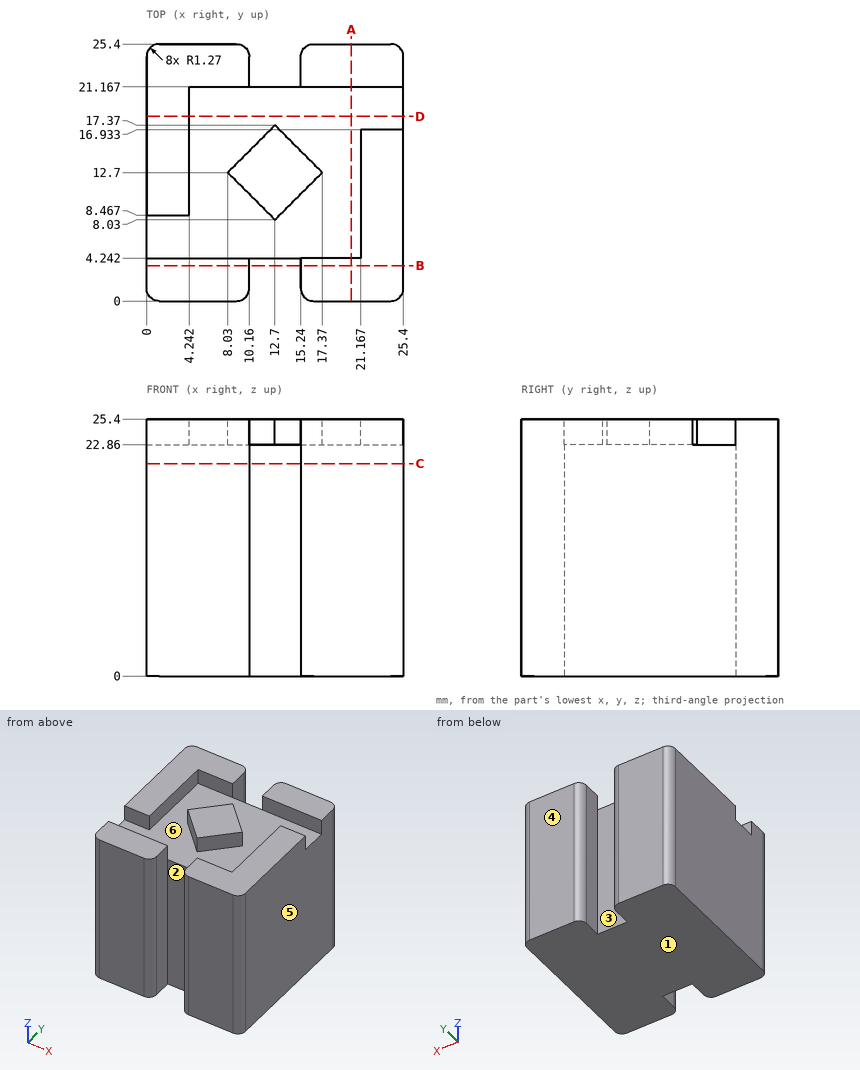
Print and shaded views of the part. All mm, measured from the part's lowest x, y and z. A direction names the side the tool comes from. Coordinates: 2 decimals unless noted, no trailing zeros. Order: outer loops, then holes, each group sorted by start corner. A loop starts at its lowest first (then second) coordinate and runs counter-clockwise, first axis right, second up. Notation, with made-up numbers: (51.5, 46) - (55.5, 46) arc R34 ccw to (55.5, 77) - close; hole circle Ø8 at (69.25, 13). An arc over 180 degrees is marked (long way). Put each result on its own line as item: value.
1. Saw through at C-C (z = 21). Write the cut outline in (x, y), and give its area (3 significant figures).
Answer sheet:
outline: (0, 1.27) arc R1.27 ccw to (1.27, 0) - (8.89, 0) arc R1.27 ccw to (10.16, 1.27) - (10.16, 4.24) - (15.24, 4.24) - (15.24, 1.27) arc R1.27 ccw to (16.51, 0) - (24.13, 0) arc R1.27 ccw to (25.4, 1.27) - (25.4, 24.13) arc R1.27 ccw to (24.13, 25.4) - (16.51, 25.4) arc R1.27 ccw to (15.24, 24.13) - (15.24, 21.17) - (10.16, 21.17) - (10.16, 24.13) arc R1.27 ccw to (8.89, 25.4) - (1.27, 25.4) arc R1.27 ccw to (0, 24.13) - close
area: 599 mm^2
2. Drop flat-ended pins along their axis: P1, Ø0.8, axis at x = 2.5, z = 24.5, coming from the -Y side; P2, Ø1.5, axis at x = 8, y = 14.5, coming from the +Z side; P3, Ø0.8, axis at y = 17.5, z = 24.5, coming from the +X side; P4, Ø4, axis at x = 13, z = 8, coming from the -Y side. Give the stop position or say it passes through.
Answer sheet:
P1: stops at y = 0
P2: stops at z = 22.86
P3: stops at x = 12.97
P4: stops at y = 4.24
3. Saw through at D-D (y = 18.25). Write the cut outline in (x, z), and give its area (3 significant figures).
Answer sheet:
outline: (0, 0) - (25.4, 0) - (25.4, 22.86) - (4.24, 22.86) - (4.24, 25.4) - (0, 25.4) - close
area: 591 mm^2
4. Saw through at A-A (x = 20.25). Write the cut outline in (y, z).
Answer sheet:
outline: (0, 0) - (25.4, 0) - (25.4, 25.4) - (21.17, 25.4) - (21.17, 22.86) - (4.24, 22.86) - (4.24, 25.4) - (0, 25.4) - close
5. Probe line 1 along X through (y, z) = (3.25, 12.5); line 2 along Y through (x, z) = (21, 23.5); line 3 along Z through (x, y) = (10.75, 17.5). List the from-to ranges inside material, lowest first. Write a range as [from, to].
Answer sheet:
line 1: x = [0, 10.16], [15.24, 25.4]
line 2: y = [0, 4.24], [21.17, 25.4]
line 3: z = [0, 22.86]
6. Saw through at B-B (y = 3.5). Write the cut outline in (x, z), and give its area (3 significant figures).
Answer sheet:
outline: (0, 0) - (10.16, 0) - (10.16, 25.4) - (0, 25.4) - close; (15.24, 0) - (25.4, 0) - (25.4, 25.4) - (15.24, 25.4) - close
area: 516 mm^2
7. Pull direction X, two halves, no side cores. Call the marked faces 3, 4, 5 and 6: pulls with the +X half, pulls with the -X half, needs draft (parallel to the pull), parting line crosses it, or undercut.
Answer sheet:
face 3: undercut
face 4: needs draft
face 5: pulls with the +X half
face 6: undercut
8. Tool access for the marked faces 1 and 2: list every direction of +Z, -Z, +X, -X, +Y, -Y with a clear straight run to the whole face (end or side of a thin tool).
Answer sheet:
face 1: -Z, +X, -X, +Y, -Y
face 2: +Z, -Z, -Y
